from build123d import *

# Parameters (mm, degrees)
BOSS_EXTRUDE1_DEPTH = 50
SKETCH4_W           = 45
SKETCH4_H           = 47.001372255
CUT_EXTRUDE2_DEPTH  = 15
SKETCH6_R           = 1.6
CUT_EXTRUDE4_DEPTH  = 5
CUT_EXTRUDE5_DEPTH  = 2.998627745
FILLET1_R           = 1


with BuildPart() as part:
    # Sketch1 → Boss-Extrude1 (new body)
    with BuildSketch(Plane.XY):
        Polygon((-10, 0), (10, 0), (10, 50), (5, 50), (-10, 3), align=None)
    extrude(amount=BOSS_EXTRUDE1_DEPTH)

    # Sketch4 → Cut-Extrude2 (cut)
    with BuildSketch(Plane.ZY.offset(10)):
        with Locations((25, 26.499313873)):
            Rectangle(SKETCH4_W, SKETCH4_H)
    extrude(amount=-CUT_EXTRUDE2_DEPTH, mode=Mode.SUBTRACT)

    # Sketch6 → Cut-Extrude4 (cut)
    with BuildSketch(Plane(origin=(10, 0, 0), x_dir=(0, 0, -1), z_dir=(1, 0, 0))):
        with Locations((-25, 25)):
            Circle(SKETCH6_R)
        with Locations((-25, 10)):
            Circle(SKETCH6_R)
        with Locations((-25, 40)):
            Circle(SKETCH6_R)
    extrude(amount=-CUT_EXTRUDE4_DEPTH, mode=Mode.SUBTRACT)

    # Sketch7 → Cut-Extrude5 (cut)
    with BuildSketch(Plane(origin=(0, 2.998627745, 0), x_dir=(1, 0, 0), z_dir=(0, 1, 0))):
        with BuildLine():
            Line((-7, -24), (3, -24))
            ThreePointArc((3, -24), (4, -25), (3, -26))
            Line((3, -26), (-7, -26))
            ThreePointArc((-7, -26), (-8, -25), (-7, -24))
        make_face()
    extrude(amount=-CUT_EXTRUDE5_DEPTH, mode=Mode.SUBTRACT)

    # Fillet1
    fillet1_edges = [part.edges().sort_by_distance(p)[0] for p in [
        (5, 2.998627745, 25),
        (-2.5, 2.998627745, 47.5),
        (-2.5, 2.998627745, 2.5),
    ]]
    fillet(fillet1_edges, radius=FILLET1_R - 0.0001)  # a hair under: the kernel refuses the full size


solid = part.part
The listing builds one solid part. Answer for the finished solid, in the listing's coordinates (mm). A direction names the side the tool comes from. Round coordinates to 2 decimals unless told otherwise and drop trailing zeros. Loops run counter-clockwise (first coordinate to the right, second up) from the corner with the lowest first, then second, coordinate; pieces in that order, holes last. Notation, with made-up numbers: M 13.5,26.5 L 55.5,26.5 A31 cw 55.5,65.5 Z; hole C 65.25,7 d3. An arc over 180 degrees is marked long. Return JSON: item names as keys, results as strings.
Q1. Find the intervals of material crossed by line 1 along Y through (x, z) = (8.95, 25); line 2 along Z through (x, y) = (-2.75, 24.5); line 3 along X through (y, z) = (34, 17.5), in increasing order. Write a range as from..to.
Results list:
{"line 1": "y = 0..8.4, 11.6..23.4, 26.6..38.4, 41.6..50", "line 2": "z = 0..2.5, 47.5..50", "line 3": "x = 5..10"}
Q2. The mould has two halves that part along Z. Classify faces 4 (the face through (2, 20, 0)), 5 (the face through (4, 2, 25)), 6 (the face through (8, 50, 25)): released by +Z, released by -Z, zero draft, split by the parting line, or undercut.
Results list:
{"face 4": "released by -Z", "face 5": "undercut", "face 6": "zero draft"}
Q3. Each of these flat-tipped pins is pushed along its axis until it touches: pin 1 Ø8 at (x, y) = (-0.5, 17.5) entering from -Z; pin 2 Ø3 at (y, z) = (12, 44) entering from -X; pin 3 Ø2.5 at (y, z) = (10, 25) entering from -X; pin 4 Ø10 at (x, z) = (-3.5, 21.5) entering from +Y. Where does it stop, or does it pass through?
Results list:
{"pin 1": "stops at z = 0", "pin 2": "stops at x = 5", "pin 3": "passes through", "pin 4": "stops at y = 3"}
Q4. Find section A-A, the plane z = 25. State how many separate pieces and enclosed holes the cut face has, plus the area to 3 significant figures.
Results list:
{"separate pieces": "5", "enclosed holes": "0", "area": "211 mm2"}
Q5. Find section C-C, the plane y = 40. Determine the outline of the cut face in (x, z), plus the area to 3 significant figures.
Results list:
{"outline": "M 1.81,0 L 10,0 L 10,23.4 L 5,23.4 L 5,2.5 L 1.81,2.5 Z; M 1.81,47.5 L 5,47.5 L 5,26.6 L 10,26.6 L 10,50 L 1.81,50 Z", "area": "250 mm2"}
Q6. Find section D-D, the plane y = 13.5. Determine the outline of the cut face in (x, z), plus the area to 3 significant figures.
Results list:
{"outline": "M -6.65,0 L 10,0 L 10,50 L -6.65,50 L -6.65,47.5 L 5,47.5 L 5,2.5 L -6.65,2.5 Z", "area": "308 mm2"}
Q7. Which of the six approach directions +Z, -Z, +X, -X, +Y, -Y give full straight-line access (tool end or side, diameter ignored) to faces 1 (the face through (1, 16, 2.5)), 2 (the face through (-8, 2, 25)), 3 (the face through (4.3, 0, 24.6))?
Results list:
{"face 1": "-X, +Y", "face 2": "+Y, -Y", "face 3": "+Z, -Z, +X, -X, -Y"}
Q8. Find section B-B, the plane x = -1.75. Determine the outline of the cut face in (y, z).
Results list:
{"outline": "M 0,0 L 28.85,0 L 28.85,2.5 L 4,2.5 A1 cw 3,3.5 L 3,24 L 0,24 Z; M 0,26 L 3,26 L 3,46.5 A1 cw 4,47.5 L 28.85,47.5 L 28.85,50 L 0,50 Z"}
